```python
from build123d import *

# Parameters (mm, degrees)
EXTRUSION1_DEPTH = 27
ESQUISSE2_W      = 20
ESQUISSE2_H      = 38
EXTRUSION2_DEPTH = 11
ESQUISSE3_R      = 18.75
EXTRUSION3_DEPTH = 58
ESQUISSE4_R      = 10
EXTRUSION4_DEPTH = 2
ESQUISSE5_R      = 3
EXTRUSION5_DEPTH = 12
CHANFREIN1_SIZE  = 1.5
CONG_1_R         = 1
ESQUISSE6_W      = 5
ESQUISSE6_H      = 1
EXTRUSION6_DEPTH = 7


with BuildPart() as part:
    # Esquisse1 → Extrusion1 (new body)
    with BuildSketch(Plane(origin=(0, 0, 0), x_dir=(1, 0, 0), z_dir=(0, 1, 0))):
        with BuildLine():
            Line((0, 0), (48.5, 0))
            ThreePointArc((48.5, 0), (56.631727984, 3.368272016), (60, 11.5))
            Line((60, 11.5), (60, 26.5))
            ThreePointArc((60, 26.5), (56.631727984, 34.631727984), (48.5, 38))
            Line((48.5, 38), (0, 38))
            Line((0, 38), (0, 0))
        make_face()
    extrude(amount=EXTRUSION1_DEPTH)

    # Esquisse2 → Extrusion2 (add)
    with BuildSketch(Plane(origin=(0, 27, 0), x_dir=(1, 0, 0), z_dir=(0, 1, 0))):
        with Locations((10, 19)):
            Rectangle(ESQUISSE2_W, ESQUISSE2_H)
    extrude(amount=EXTRUSION2_DEPTH)

    # Esquisse3 → Extrusion3 (add)
    with BuildSketch(Plane(origin=(0, 27, 0), x_dir=(1, 0, 0), z_dir=(0, 1, 0))):
        with Locations((41.25, 19)):
            Circle(ESQUISSE3_R)
    extrude(amount=EXTRUSION3_DEPTH)

    # Esquisse4 → Extrusion4 (add)
    with BuildSketch(Plane(origin=(0, 85, 0), x_dir=(1, 0, 0), z_dir=(0, 1, 0))):
        with Locations((41.25, 19)):
            Circle(ESQUISSE4_R)
    extrude(amount=EXTRUSION4_DEPTH)

    # Esquisse5 → Extrusion5 (add)
    with BuildSketch(Plane(origin=(0, 38, 0), x_dir=(1, 0, 0), z_dir=(0, 1, 0))):
        with Locations((3, 27)):
            Circle(ESQUISSE5_R)
        with Locations((3, 11)):
            Circle(ESQUISSE5_R)
    extrude(amount=EXTRUSION5_DEPTH)

    # Chanfrein1
    chanfrein1_edges = [part.edges().sort_by_distance(p)[0] for p in [
        (0, 50, -27),
        (0, 50, -11),
    ]]
    chamfer(chanfrein1_edges, length=CHANFREIN1_SIZE)

    # Congé1
    cong_1_edges = [part.edges().sort_by_distance(p)[0] for p in [
        (22.5, 85, -19),
    ]]
    fillet(cong_1_edges, radius=CONG_1_R)

    # Esquisse6 → Extrusion6 (add)
    with BuildSketch(Plane(origin=(0, 85, 0), x_dir=(1, 0, 0), z_dir=(0, 1, 0))):
        with Locations((41.25, 32.25)):
            Rectangle(ESQUISSE6_W, ESQUISSE6_H)
        with Locations((41.25, 5.75)):
            Rectangle(ESQUISSE6_W, ESQUISSE6_H)
    extrude(amount=EXTRUSION6_DEPTH)


solid = part.part
```
Input: part model. Units: mm. Frame: model coordinates. A direction names the side the tool comes from. Give positions to 0.01 mm unless a question says otherwise; leave off trailing zeros. Loops run counter-clockwise (first coordinate to the right, second up) from the corner with the lowest first, then second, coordinate; pieces in that order, holes last.
1) Line query: L1, parallel to Y at x = 10, z = -11; L2, parallel to Y at x = 20.5, z = -34.5; L3, parallel to Z at x = 55, y = 79. Output: solid intervals per line, ascending.
A:
L1: y = 0 to 38
L2: y = 0 to 27
L3: z = -31.75 to -6.25
2) Section query C-C on y = 72.5. Return the cut outline in (x, z), and give its area (3 significant figures).
A:
outline: circle Ø37.5 at (41.25, -19)
area: 1,100 mm2
3) Reachability of faces 5 (the flat face through (41, 88, -32.75)), 6 (the flat face through (20, 32, -19)), 7 (the flat face through (3, 50, -11)) from +Z, -Z, +X, -X, +Y, -Y: full face, straight path, thin tool, end or side. Return the list, or none.
A:
face 5: -Z, +X, -X, +Y
face 6: +Z, -Z, +Y
face 7: +Z, -Z, -X, +Y
4) Section query D-D on x = 41.25. Return the cut outline in (y, z).
A:
outline: (0, -38) - (27, -38) - (27, -37.75) - (84, -37.75) arc R1 ccw to (85, -36.75) - (85, -32.75) - (92, -32.75) - (92, -31.75) - (85, -31.75) - (85, -29) - (87, -29) - (87, -9) - (85, -9) - (85, -6.25) - (92, -6.25) - (92, -5.25) - (85, -5.25) - (85, -1.25) arc R1 ccw to (84, -0.25) - (27, -0.25) - (27, 0) - (0, 0) - close
5) Contact query for flat-ended pins moving along their axis: pin 1 (1.5 mm diameter, centred on x = 39.5, y = 28.5, fed in from +Z); pin 2 (2.5 mm diameter, centred on x = 42.5, y = 87.5, fed in from +Z); pin 3 (1.1 mm diameter, centred on y = 87.5, z = -5.5, fed in from -X). Output: stop coordinate, or through.
A:
pin 1: stops at z = -0.28
pin 2: stops at z = -5.25
pin 3: stops at x = 38.75
6) Mould query, pull axis Z, two halves, no side actions, for faces 1 (the cylindrical face through (0.6, 43.2, -25.2)), 2 (the flat face through (41, 88, -31.75)), 3 (the cylindrical face through (56.72, 13.31, -34.54)), 4 (the cylindrical face through (56.54, 13.31, -3.28)). Classes: released by +Z, released by -Z, zero draft, split by the parting line, or undercut.
A:
face 1: undercut
face 2: undercut
face 3: released by -Z
face 4: released by +Z
7) Section query A-A on y = 29.5. Return the cut outline in (x, z).
A:
outline: (0, -38) - (20, -38) - (20, 0) - (0, 0) - close; circle Ø37.5 at (41.25, -19)
8) Section query B-B on x = 3. Return the cut outline in (y, z).
A:
outline: (0, -38) - (38, -38) - (38, -30) - (48.5, -30) - (50, -28.5) - (50, -25.5) - (48.5, -24) - (38, -24) - (38, -14) - (48.5, -14) - (50, -12.5) - (50, -9.5) - (48.5, -8) - (38, -8) - (38, 0) - (0, 0) - close
